Verification items for the finished model (mm, model axes). A direction names the side the tool comes from. Give positions to 0.01 mm unless a question says otherwise; leave off trailing zeros. Loops run counter-clockwise (first coordinate to the right, second up) from the corner with the lowest first, then second, coordinate; pieces in that order, holes last. Notation, with made-up numbers: (2.5, 86.25) -> (26.5, 86.25) arc R7 ccw to (26.5, 99.25) -> close; hole circle Ø8 at (-14.5, 17). An arc over 180 degrees is marked (long way). Answer in a Markdown table with one row per item. Add a question column.
Q1. Gauge pin test, flat ends, axial feed: P1, Ø2, axis at y = 64.78, z = -16.1, coming from the -X side; P2, Ø5, axis at y = 42.05, z = -2.98, coming from the -X side; P3, Ø1.5, axis at x = -38.5, z = -1, coming from the +Y side; P4, Ø1.5, axis at x = -12.5, z = -12.5, coming from the -Y side. Record the tip position at first contact, or that the pin passes through.
Q2. Section check A-A on y = 42.05. Enter the section's corners in (x, z), and give its area (3 significant figures).
Q3. Release check for a two-part mould opening along X. For faces 4 (the face through (0, 29, -3)), 5 (the face through (-1.01, 40.41, -2.12)), 6 (the face through (-43.25, 1.01, -15.53)) record: pulls with the +X half, pulls with the -X half, needs draft (parallel to the pull), parting line crosses it, or undercut.
Q4. Material ranges on probe 1 along X at (y, z) = (38, 13); probe 2 along Y at (x, z) = (-29, 3.5), recorded low to high.
Q5. Set-up check for faces 1 (the face through (-1, 16, -21.976)), 2 (the face through (-26.25, 1.01, 9.37)), 3 (the face through (-24, 2, -3)): record each of +Z, -Z, +X, -X, +Y, -Y from which the full face is reachable in a straight line by a thin tool's end or side.
Q6. Section check C-C on y = 61. Enter the section's corners in (x, z), and give its area (3 significant figures).
Q7. Section check D-D on x = -4. Enter the section's corners in (y, z).
Q8. Section check B-B on z = 11. Enter the section's corners in (x, y).
```python
from build123d import *

# Parameters (mm, degrees)
SKETCH1_W           = 45.35
SKETCH1_H           = 38
BOSS_EXTRUDE1_DEPTH = 2
SKETCH2_W           = 2
SKETCH2_H           = 38
BOSS_EXTRUDE2_DEPTH = 74.25
SKETCH3_R           = 10.2
SKETCH3_R_2         = 1.85
CUT_EXTRUDE1_DEPTH  = 50
CUT_EXTRUDE2_DEPTH  = 46.35
CUT_EXTRUDE3_DEPTH  = 3


with BuildPart() as part:
    # Sketch1 → Boss-Extrude1 (new body)
    with BuildSketch(Plane(origin=(0, 0, 0), x_dir=(1, 0, 0), z_dir=(0, 1, 0))):
        with Locations((-22.675, 2.976284585)):
            Rectangle(SKETCH1_W, SKETCH1_H)
    extrude(amount=BOSS_EXTRUDE1_DEPTH)

    # Sketch2 → Boss-Extrude2 (add)
    with BuildSketch(Plane(origin=(0, 2, 0), x_dir=(1, 0, 0), z_dir=(0, 1, 0))):
        with Locations((-1, 2.976284585)):
            Rectangle(SKETCH2_W, SKETCH2_H)
    extrude(amount=BOSS_EXTRUDE2_DEPTH)

    # Sketch3 → Cut-Extrude1 (cut)
    with BuildSketch(Plane.ZY.offset(2)):
        with Locations((-2.976284585, 57.2)):
            Circle(SKETCH3_R)
        with Locations((-16.096569452, 64.775)):
            Circle(SKETCH3_R_2)
        with Locations((10.144000282, 64.775)):
            Circle(SKETCH3_R_2)
        with Locations((-2.976284585, 42.05)):
            Circle(SKETCH3_R_2)
    extrude(amount=-CUT_EXTRUDE1_DEPTH, mode=Mode.SUBTRACT)

    # Sketch14 → Cut-Extrude2 (cut, through all)
    with BuildSketch(Plane(origin=(0, 0, 0), x_dir=(0, 0, -1), z_dir=(1, 0, 0))):
        with BuildLine():
            Line((-16.023715415, 57.2), (-16.023715415, 90.282409195))
            Line((-16.023715415, 90.282409195), (21.976284585, 90.282409195))
            Line((21.976284585, 90.282409195), (21.976284585, 57.2))
            ThreePointArc((21.976284585, 57.2), (2.976284585, 76.2), (-16.023715415, 57.2))
        make_face()
    extrude(amount=-CUT_EXTRUDE2_DEPTH, mode=Mode.SUBTRACT)

    # Sketch15 → Cut-Extrude3 (cut, through all)
    with BuildSketch(Plane(origin=(0, 2, 0), x_dir=(1, 0, 0), z_dir=(0, 1, 0))):
        with BuildLine():
            Line((-30.75, -13.973715415), (-38.75, -13.973715415))
            ThreePointArc((-38.75, -13.973715415), (-43.25, -9.473715415), (-38.75, -4.973715415))
            Line((-38.75, -4.973715415), (-30.75, -4.973715415))
            ThreePointArc((-30.75, -4.973715415), (-26.25, -9.473715415), (-30.75, -13.973715415))
        make_face()
        with BuildLine():
            Line((-30.75, 19.926284585), (-38.75, 19.926284585))
            ThreePointArc((-38.75, 19.926284585), (-43.25, 15.426284585), (-38.75, 10.926284585))
            Line((-38.75, 10.926284585), (-30.75, 10.926284585))
            ThreePointArc((-30.75, 10.926284585), (-26.25, 15.426284585), (-30.75, 19.926284585))
        make_face()
    extrude(amount=-CUT_EXTRUDE3_DEPTH, mode=Mode.SUBTRACT)


solid = part.part
```
Taken from the geometry:
| question | item | result |
|---|---|---|
| 1 | P1 | passes through |
| 1 | P2 | stops at x = -2 |
| 1 | P3 | stops at y = 2 |
| 1 | P4 | stops at y = 0 |
| 2 | outline | (-2, -21.98) -> (0, -21.98) -> (0, -4.83) -> (-2, -4.83) -> close; (-2, -1.13) -> (0, -1.13) -> (0, 16.02) -> (-2, 16.02) -> close |
| 2 | area | 68.6 mm² |
| 3 | face 4 | pulls with the +X half |
| 3 | face 5 | needs draft |
| 3 | face 6 | undercut |
| 4 | probe 1 | x = -2 to 0 |
| 4 | probe 2 | y = 0 to 2 |
| 5 | face 1 | -Z, +X, -X, +Y, -Y |
| 5 | face 2 | +Y, -Y |
| 5 | face 3 | +Z, -Z, -X, +Y |
| 6 | outline | (-2, -21.59) -> (0, -21.59) -> (0, -12.44) -> (-2, -12.44) -> close; (-2, 6.49) -> (0, 6.49) -> (0, 15.64) -> (-2, 15.64) -> close |
| 6 | area | 36.6 mm² |
| 7 | outline | (0, -21.98) -> (2, -21.98) -> (2, 16.02) -> (0, 16.02) -> close |
| 8 | outline | (-45.35, 0) -> (-42.98, 0) -> (-42.98, 2) -> (-45.35, 2) -> close; (-26.52, 0) -> (0, 0) -> (0, 63.13) -> (-2, 63.13) -> (-2, 2) -> (-26.52, 2) -> close; (-2, 66.42) -> (0, 66.42) -> (0, 70.07) -> (-2, 70.07) -> close |
